Autodesk Inventor part; units mm, degrees
ref_plane "YZ Plane" through (0, 0, 0) normal (1, 0, 0) x (0, 1, 0)
ref_plane "XZ Plane" through (0, 0, 0) normal (0, 1, 0) x (-1, 0, 0)
ref_plane "XY Plane" through (0, 0, 0) normal (0, 0, 1) x (1, 0, 0)
sketch "Sketch1" plane through (0, 0, 0) normal (0, 1, 0) x (-1, 0, 0)
  line L0 (0, 0) -> (92.5, 0)
  line L1 (92.5, -97.5) -> (0, -97.5)
  line L2 (0, -97.5) -> (0, 0)
  line L3 (92.5, 0) -> (69, 0)
  line L4 (69, 0) -> (69, -97.5)
  line L5 (92.5, -97.5) -> (69, -97.5)
  line L6 (0, -97.5) -> (13, -97.5)
  line L7 (13, -97.5) -> (13, -89.5)
  line L8 (13, -89.5) -> (0, -89.5)
  line L9 (0, -89.5) -> (0, -97.5)
  line L10 (0, 0) -> (13, 0)
  line L11 (13, 0) -> (13, -8)
  line L12 (13, -8) -> (0, -8)
  line L13 (0, -8) -> (0, 0)
  point P0 (69, -97.5)
  dimension "d0" = 92.5
  dimension "d1" = 97.5
  dimension "d4" = 13
  dimension "d5" = 8
  dimension "d24" = 69
extrude "Extrusion1" add sketch "Sketch1" along normal blind 2 contours L0 L4 L1 L7 L8 L2 L12 L11
sketch "Sketch2" plane through (0, 2, 0) normal (0, 1, 0) x (1, 0, 0)
  circle A0 centre (-2.2, 10.15) radius 1.6421
  circle A1 centre (-2.2, 48.75) radius 1.6421
  circle A2 centre (-2.2, 87.35) radius 1.6421
  point P0 (0, 0)
hole "Hole1" at (-2.2, 2, -10.15) at (-2.2, 2, -48.75) at (-2.2, 2, -87.35) direction (0, -1, 0) diameter 2.459 end through all countersink diameter 3.6 countersink angle 90
sketch "Sketch3" plane through (0, 0, 0) normal (0, -1, 0) x (1, 0, 0)
  line L0 (-13, -97.5) -> (-69, -97.5) construction
  line L1 (-13, -89.5) -> (-13, -97.5) construction
  line L2 (0, -8) -> (0, -89.5) construction
  line L3 (0, -48.75) -> (-69, -48.75) construction
  line L4 (-69, -97.5) -> (-69, 0) construction
  point P0 (-13, 0)
  point P1 (-16, -94.5)
  point P2 (-38, -94.5)
  point P3 (-16, -3)
  point P4 (-38, -3)
  dimension "d25" = 3
  dimension "d26" = 3
  dimension "d27" = 22
hole "Hole2" at (-16, 0, -94.5) at (-38, 0, -94.5) at (-16, 0, -3) at (-38, 0, -3) direction (0, 1, 0) diameter 3.4 end through all countersink diameter 6.3 countersink angle 90
properties part number "Blacha" material "Steel"
Here's how the part is built. I have some questions about the finished solid (model axes, mm). A direction names the side the tool comes from. Coordinates: 2 decimals unless noted, no trailing zeros. Loops run counter-clockwise (first coordinate to the right, second up) from the corner with the lowest first, then second, coordinate; pieces in that order, holes last. Notation, with made-up numbers: (65, -34.75) -> (101, -34.75) arc R32 ccw to (101, 1.25) -> close; hole circle Ø6 at (46, 58.5). An arc over 180 degrees is marked (long way). Return JSON: item names as keys, results as strings.
1) If we section it at C-C, the plane z = -3: Write out the boundary of the cut face in (x, y), then the cut area to 3 significant figures.
Results below:
{"outline": "(-69, 0) -> (-41.15, 0) -> (-39.7, 1.45) -> (-39.7, 2) -> (-69, 2) -> close; (-36.3, 1.45) -> (-34.85, 0) -> (-19.15, 0) -> (-17.7, 1.45) -> (-17.7, 2) -> (-36.3, 2) -> close; (-14.3, 1.45) -> (-13, 0.15) -> (-13, 2) -> (-14.3, 2) -> close", "area": "94.2 mm²"}
2) Thinking about a two-plate mould opening in X: for faces 4 (the face through (-13, 1, -4)), 5 (the face through (-1.729, 0.705, -9.014)), 6 (the face through (-34, 2, -48)), which applies, +X half, -X half, draft (parallel to the pull), parting line (faces both ways), or undercut?
Results below:
{"face 4": "+X half", "face 5": "undercut", "face 6": "draft"}
3) Will these pins go through, and if not, where does the flat tip stop? pin 1 (2 mm diameter, centred on x = -2.2, z = -10.15, fed in from +Y); pin 2 (4 mm diameter, centred on x = -31.5, z = -54, fed in from -Y); pin 3 (1 mm diameter, centred on y = 0.5, z = -5, fed in from +X); pin 4 (0.6 mm diameter, centred on x = -8.5, y = 0.5, fed in from -Z).
Results below:
{"pin 1": "through", "pin 2": "y = 0", "pin 3": "x = -13", "pin 4": "z = -89.5"}
4) If we section it at A-A, the plane x = -16: Write out the boundary of the cut face in (y, z), then the cut area to 3 significant figures.
Results below:
{"outline": "(0, -91.35) -> (1.45, -92.8) -> (2, -92.8) -> (2, -4.7) -> (1.45, -4.7) -> (0, -6.15) -> close; (0.15, -97.5) -> (2, -97.5) -> (2, -96.2) -> (1.45, -96.2) -> close; (0.15, 0) -> (1.45, -1.3) -> (2, -1.3) -> (2, 0) -> close", "area": "177 mm²"}
5) I need wall thicknesses on line 1 (Z direction, x = -38, y = 1.85); line 2 (X direction, y = 1.65, z = -3); line 3 (Z direction, x = -2.2, y = 0.8). Which ranges of each line are inside material? Lowest first, please. Write a range as from..to.
Results below:
{"line 1": "-97.5..-96.2, -92.8..-4.7, -1.3..0", "line 2": "-69..-39.7, -36.3..-17.7, -14.3..-13", "line 3": "-89.5..-88.58, -86.12..-49.98, -47.52..-11.38, -8.92..-8"}
6) If we section it at B-B, the plane y = 0.55: Write out the boundary of the cut face in (x, z).
Results below:
{"outline": "(-69, -97.5) -> (-13, -97.5) -> (-13, -89.5) -> (0, -89.5) -> (0, -8) -> (-13, -8) -> (-13, 0) -> (-69, 0) -> close; hole circle Ø5.2 at (-38, -94.5); hole circle Ø5.2 at (-38, -3); hole circle Ø5.2 at (-16, -94.5); hole circle Ø5.2 at (-16, -3); hole circle Ø2.46 at (-2.2, -87.35); hole circle Ø2.46 at (-2.2, -48.75); hole circle Ø2.46 at (-2.2, -10.15)"}
7) For faces 1 (the face through (-13, 1, -94)), 2 (the face through (-16.07, 1.73, -92.8)), 3 (the face through (-7, 1, -8)), which set-ups out of +Z, -Z, +X, -X, +Y, -Y let a thin tool reach every point of the face, with its end or its side?
Results below:
{"face 1": "-Z, +X, +Y, -Y", "face 2": "+Y, -Y", "face 3": "+Z, +X, +Y, -Y"}
8) If we section it at D-D, the plane x = -2.2: Write out the boundary of the cut face in (y, z), then the cut area to 3 significant figures.
Results below:
{"outline": "(0, -89.5) -> (2, -89.5) -> (2, -89.15) -> (1.43, -88.58) -> (0, -88.58) -> close; (0, -86.12) -> (1.43, -86.12) -> (2, -85.55) -> (2, -50.55) -> (1.43, -49.98) -> (0, -49.98) -> close; (0, -47.52) -> (1.43, -47.52) -> (2, -46.95) -> (2, -11.95) -> (1.43, -11.38) -> (0, -11.38) -> close; (0, -8.92) -> (1.43, -8.92) -> (2, -8.35) -> (2, -8) -> (0, -8) -> close", "area": "147 mm²"}
